Here's the drawing with two shaded views (mm, measured from the low corner). I have some questions. Give positions to 0.01 mm unless a question says otherwise; leave off trailing zeros. Loops run counter-clockwise (first coordinate to the right, second up) from the corner with the lowest first, then second, coordinate; pieces in that order, holes last. Notation, with made-up numbers: (45, -11) - (92, -11) arc R24 cw to (92, 26) - close; hole circle Ø4 at (49.25, 40.5). An arc over 180 degrees is marked (long way). Use a Markdown table: item, result. Add a question column.
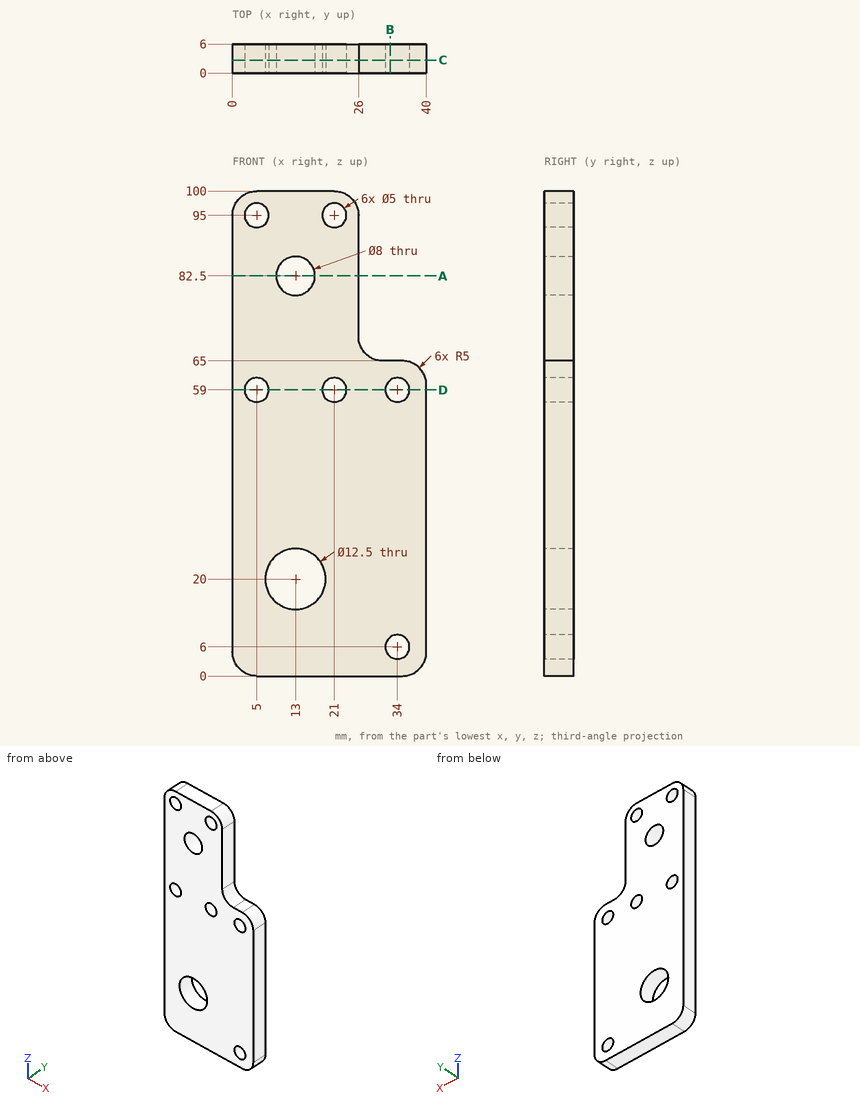
1. Suppose I cut it at C-C (y = 2.65). State how many separate pieces and enclosed holes the cut face has, and give its area (3 significant figures).
2. Suppose I cut it at D-D (z = 59). List the corners of the cut face in (x, y) for me.
3. Will these pins go through, and if not, where does the flat tip stop? P1, Ø1.8, axis at y = 3.5, z = 86.5, coming from the +X side; P2, Ø6, axis at x = 5, z = 95, coming from the -Y side; P3, Ø1.5, axis at x = 23, y = 2.5, coming from the +Z side.
4. Suppose I cut it at B-B (x = 32.5). List the corners of the cut face in (y, z) for me.
5. Suppose I cut it at A-A (z = 82.5). List the corners of the cut face in (x, y) for me.
6. Please list where these lines run through material, in increasing order: line 1 along Z through (x, y) = (13, 3.15); line 2 along Z through (x, y) = (5, 4.05); line 3 along X through (y, z) = (2.8, 59). Write a range as [from, to].
Results below:
| question | item | result |
|---|---|---|
| 1 | separate pieces | 1 |
| 1 | enclosed holes | 8 |
| 1 | area | 3,200 mm² |
| 2 | outline | (0, 0) - (2.5, 0) - (2.5, 6) - (0, 6) - close; (7.5, 0) - (18.5, 0) - (18.5, 6) - (7.5, 6) - close; (23.5, 0) - (31.5, 0) - (31.5, 6) - (23.5, 6) - close; (36.5, 0) - (40, 0) - (40, 6) - (36.5, 6) - close |
| 3 | P1 | x = 26 |
| 3 | P2 | y = 0 |
| 3 | P3 | z = 99.84 |
| 4 | outline | (0, 0) - (6, 0) - (6, 4) - (0, 4) - close; (0, 8) - (6, 8) - (6, 57) - (0, 57) - close; (0, 61) - (6, 61) - (6, 65) - (0, 65) - close |
| 5 | outline | (0, 0) - (9, 0) - (9, 6) - (0, 6) - close; (17, 0) - (26, 0) - (26, 6) - (17, 6) - close |
| 6 | line 1 | [0, 13.75], [26.25, 78.5], [86.5, 100] |
| 6 | line 2 | [0, 56.5], [61.5, 92.5], [97.5, 100] |
| 6 | line 3 | [0, 2.5], [7.5, 18.5], [23.5, 31.5], [36.5, 40] |
